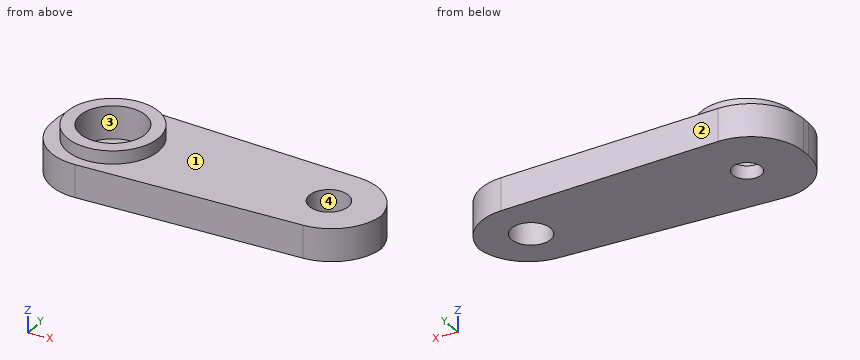
from build123d import *

# Parameters (mm, degrees)
F0_R        = 2.5
F0_R_2      = 1.5
F1_DEPTH    = 2.5
F2_T1_DEPTH = 21.7159936051
F2_T3_DEPTH = 23.3159936051
F3_R        = 3.5
F3_R_2      = 2.5
F4_DEPTH    = 1
F5_R        = 2.5
F5_R_2      = 1.1
F6_DEPTH    = 1


# Not quite as in the source:
# - a fillet or chamfer that OpenCascade refuses, or shapes differently, is made with other operations: its cross-section is extruded or revolved along the edge and cut away or added


with BuildPart() as f1:
    # F0 (on Top) → F1 (new body)
    with BuildSketch(Plane.XY):
        Polygon((25, -12), (0, -11), (0, -20), (25, -19), align=None)
        with Locations((4.5, -15.5)):
            Circle(F0_R, mode=Mode.SUBTRACT)
        with Locations((21, -15.5)):
            Circle(F0_R_2, mode=Mode.SUBTRACT)
    extrude(amount=F1_DEPTH)

    # F2: fillet of radius 4 on 4 edges, made by hand

    # F2_s2 → F2_t1 (cut)
    with BuildSketch(Plane.XY.offset(-9.6079968026)):
        with BuildLine():
            ThreePointArc((21.1598721534, -11.8463948861), (23.8843966972, -13.0718712966), (25, -15.843198721))
            Line((25, -15.843198721), (25, -12))
            Line((25, -12), (21.1598721534, -11.8463948861))
        make_face()
        with BuildLine():
            ThreePointArc((21.1598721534, -19.1536051139), (23.8843966972, -17.9281287034), (25, -15.156801279))
            Line((25, -15.156801279), (25, -19))
            Line((25, -19), (21.1598721534, -19.1536051139))
        make_face()
    extrude(amount=F2_T1_DEPTH, mode=Mode.SUBTRACT)

    # F2_s4 → F2_t3 (cut)
    with BuildSketch(Plane.XY.offset(-10.4079968026)):
        with BuildLine():
            ThreePointArc((4.1598721534, -11.1663948861), (1.2286725756, -12.2788020238), (0, -15.163198721))
            Line((0, -15.163198721), (0, -11))
            Line((0, -11), (4.1598721534, -11.1663948861))
        make_face()
        with BuildLine():
            ThreePointArc((0, -15.836801279), (1.2286725756, -18.7211979762), (4.1598721534, -19.8336051139))
            Line((4.1598721534, -19.8336051139), (0, -20))
            Line((0, -20), (0, -15.836801279))
        make_face()
    extrude(amount=F2_T3_DEPTH, mode=Mode.SUBTRACT)

    # F3 (on face) → F4 (join)
    with BuildSketch(Plane.XY.offset(2.5)):
        with Locations((4.5, -15.5)):
            Circle(F3_R)
        with Locations((4.5, -15.5)):
            Circle(F3_R_2, mode=Mode.SUBTRACT)
    extrude(amount=F4_DEPTH)

    # F5 (on Top) → F6 (join)
    with BuildSketch(Plane.XY):
        with Locations((4.5, -15.5)):
            Circle(F5_R)
        with Locations((4.5, -15.5)):
            Circle(F5_R_2, mode=Mode.SUBTRACT)
    extrude(amount=F6_DEPTH)


solid = f1.part
Can you work these out from the model? Positions are in its coordinate system, mm. Face numbers are marked on the shaded views. Coordinates: 2 decimals unless noted, no trailing zeros. Loops run counter-clockwise (first coordinate to the right, second up) from the corner with the lowest first, then second, coordinate; pieces in that order, holes last. Notation, with made-up numbers: M 23,5.25 L 29,5.25 A32 ccw 29,34.25 Z; hole C 53.5,-29 d3. An arc over 180 degrees is marked long. Answer as CSV lines item,"result". Start each with the question number.
1. Suppose I cut it at D-D, the plane x = 20.75. List the corners of the cut face in (y, z) for me.
2. Thinking about a two-plate mould opening in Y: for the marked faces 1, 2, 3 and 4, which applies, +Y half, -Y half, draft (parallel to the pull), parting line (faces both ways), or undercut?
3. Suppose I cut it at B-B, the plane z = 2.85. List the corners of the cut face in (x, y) for me, plus the area to 3 significant figures.
4. If I drill on probe 1 along X at (y, z) = (-14.5, 1.6); probe 2 along X at (y, z) = (-15.75, 1.2); probe 3 along Z at (x, y) = (4.75, -17), over which ranges is the centre line in solid material (lowest first)? Write a range as [from, to].
5. Suppose I cut it at A-A, the plane x = 4.5. List the corners of the cut face in (y, z) for me, plus the area to 3 significant figures.
6. Suppose I cut it at C-C, the plane y = -12.75. List the corners of the cut face in (x, z) for me, plus the area to 3 significant figures.
7. For pin 1 Ø1.5 at (y, z) = (-18.5, 2.5) entering from -X; pin 2 Ø1.8 at (x, y) = (21, -15.5) entering from -Z; pin 3 Ø3 at (x, y) = (4.5, -15.5) entering from -Z; pin 4 Ø1.5 at (y, z) = (-17.5, 1) entering from -X, each with a flat end and sliding along its axis, tell me the tip position at first contact or that it passes through.
Output:
1,outline,"M -19.17,0 L -16.98,0 L -16.98,2.5 L -19.17,2.5 Z; M -14.02,0 L -11.83,0 L -11.83,2.5 L -14.02,2.5 Z"
2,face 1,"draft"
2,face 2,"+Y half"
2,face 3,"undercut"
2,face 4,"undercut"
3,outline,"C 4.5,-15.5 d7; hole C 4.5,-15.5 d5"
3,area,"18.8 mm^2"
4,probe 1,"x = [0.06, 2.21], [6.79, 19.88], [22.12, 24.77]"
4,probe 2,"x = [0, 2.01], [6.99, 19.52], [22.48, 24.96]"
4,probe 3,"z = [0, 1]"
5,outline,"M -19.82,0 L -16.6,0 L -16.6,1 L -18,1 L -18,3.5 L -19,3.5 L -19,2.5 L -19.82,2.5 Z; M -14.4,0 L -11.18,0 L -11.18,2.5 L -12,2.5 L -12,3.5 L -13,3.5 L -13,1 L -14.4,1 Z"
5,area,"13.9 mm^2"
6,outline,"M 0.81,0 L 23.54,0 L 23.54,2.5 L 6.67,2.5 L 6.67,3.5 L 2.33,3.5 L 2.33,2.5 L 0.81,2.5 Z"
6,area,"61.1 mm^2"
7,pin 1,"stops at x = 0.49"
7,pin 2,"passes through"
7,pin 3,"stops at z = 0"
7,pin 4,"stops at x = 0.11"
